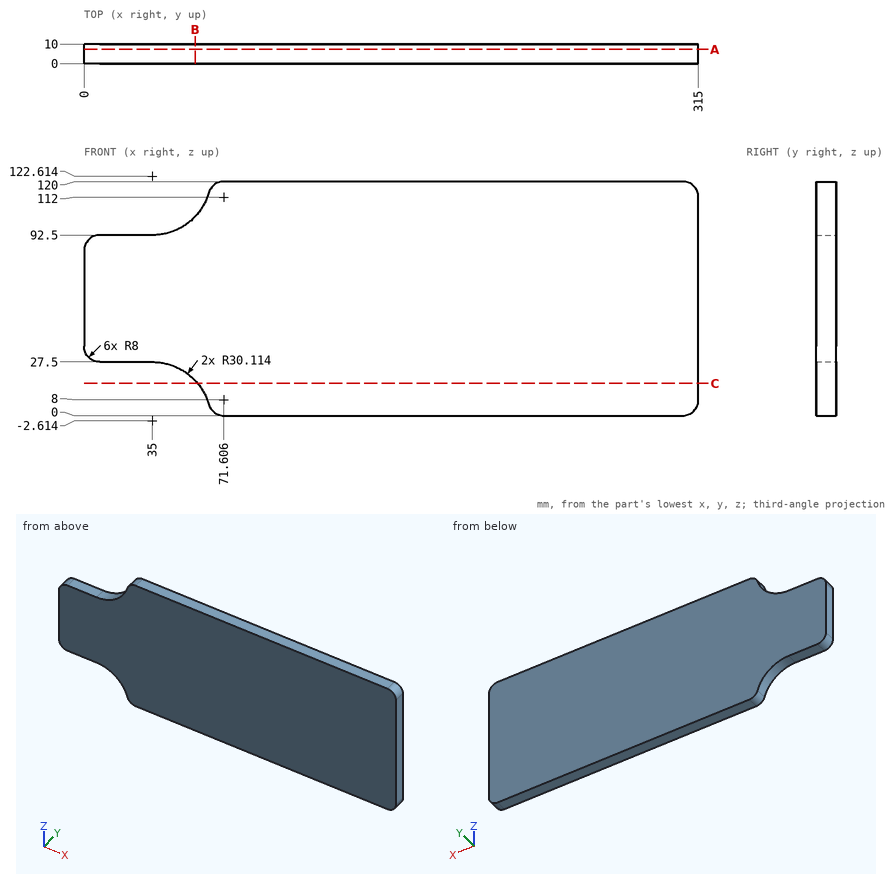
Job drawing, mm, ordinate dimensions from the low corner. One solid piece. Round coordinates to 2 decimals unless told otherwise and drop trailing zeros. Loops run counter-clockwise (first coordinate to the right, second up) from the corner with the lowest first, then second, coordinate; pieces in that order, holes last. Notation, with made-up numbers: M 87.25,23 L 132.25,23 A18 ccw 132.25,38 Z; hole C 74.5,10.5 d2. An arc over 180 degrees is marked long. Answer as CSV lines item,"result".
1. Cut at C-C on z = 16.5. Write the cut outline in (x, y).
Resolved:
outline,"M 58.27,0 L 315,0 L 315,10 L 58.27,10 Z"
2. Flat gauge pins, fed straight in: P1, Ø6, axis at x = 44.5, y = 8.5, coming from the -Z side; P2, Ø5, axis at x = 15.5, y = 2.5, coming from the +Z side; P3, Ø4, axis at y = 2, z = 98.5, coming from the -X side (1 decimal). Where does each tip first touch, or does it go through?
Resolved:
P1,"stops at z = 24.78"
P2,"stops at z = 92.5"
P3,"stops at x = 50"
3. Cut at A-A on y = 7.25. Write the cut outline in (x, z), then the cut area to 3 significant figures.
Resolved:
outline,"M 0,35.5 A8 ccw 8,27.5 L 35,27.5 A30.11 cw 63.92,5.77 A8 ccw 71.61,0 L 307,0 A8 ccw 315,8 L 315,112 A8 ccw 307,120 L 71.61,120 A8 ccw 63.92,114.23 A30.11 cw 35,92.5 L 8,92.5 A8 ccw 0,84.5 Z"
area,"34,500 mm²"
4. Wall check: probe 1 along X at (y, z) = (3, 85) (1 decimal); probe 2 along X at (y, z) = (8.75, 34.5); probe 3 along Z at (x, y) = (44, 6.25). Give the ranges that are in metal, low to high. Write a range as [from, to].
Resolved:
probe 1,"x = [0, 315]"
probe 2,"x = [0.06, 315]"
probe 3,"z = [26.12, 93.88]"
5. Cut at B-B on x = 57. Write the cut outline in (y, z).
Resolved:
outline,"M 0,17.95 L 10,17.95 L 10,102.05 L 0,102.05 Z"
